```python
from build123d import *

# Parameters (mm, degrees)
BOSS_EXTRUDE1_DEPTH = 2.667
CUT_EXTRUDE1_DEPTH  = 290.953060218


with BuildPart() as part:
    # Sketch1 → Boss-Extrude1 (new body)
    with BuildSketch(Plane(origin=(0, 0, 0), x_dir=(0, 0, -1), z_dir=(1, 0, 0))):
        Polygon((0, 0), (168.275, 0), (251.079, 145), (161.163, 145), align=None)
    extrude(amount=BOSS_EXTRUDE1_DEPTH)

    # Sketch2 → Cut-Extrude1 (cut, through all)
    with BuildSketch(Plane.ZY):
        with BuildLine():
            Line((-38.268496776, -3.7413e-05), (1.603827089, -0.136652983))
            Line((1.603827089, -0.136652983), (-7.656991971, 9.482815094))
            Line((-7.656991971, 9.482815094), (-10.613049229, 9.482815094))
            add(Edge.make_bspline(
                [(-9.096096952, 6.965105301), (-9.056659473, 7.842017541), (-9.649957621, 8.686611456), (-10.613049229, 9.482815094)],
                knots=[0.095003114, 0.095003114, 0.095003114, 0.095003114, 0.122643686, 0.122643686, 0.122643686, 0.122643686], degree=3))
            add(Edge.make_bspline(
                [(-20.479171235, 1.104059742), (-19.78420669, 1.190866413), (-14.294371688, 1.692059126), (-9.186269713, 4.960068489), (-9.096096952, 6.965105301)],
                knots=[0, 0, 0, 0, 0.031803671, 0.095003114, 0.095003114, 0.095003114, 0.095003114], degree=3))
            add(Edge.make_bspline(
                [(-38.268496776, -3.7413e-05), (-29.333639406, -0.001953509), (-20.479171235, 1.104059742)],
                knots=[0, 0, 0, 1, 1, 1], degree=2))
        make_face()
    extrude(amount=-CUT_EXTRUDE1_DEPTH, mode=Mode.SUBTRACT)


solid = part.part
```
For this review, take the finished solid that the model builds, in its own axes (mm). Coordinates: 2 decimals unless noted, no trailing zeros. Write each loop counter-clockwise with the first axis right and the second up, starting at its lowest first coordinate (ties: lowest second). Pieces come first, ordered by that corner, then holes. Notation, with made-up numbers: (33.5, 70) - (57.5, 70) arc R8 ccw to (57.5, 79) - close; hole circle Ø11 at (-15, -22.75). An arc over 180 degrees is marked (long way). Answer in a Markdown table with one row per item. Add a question column.
Q1. For P1, Ø1.5, axis at x = 0.5, z = -138.5, coming from the +Y side, flat-tipped, find the tip position at first contact; note if it passes through.
Q2. For probe 1 along Z at (x, y) = (2.15, 138); probe 2 along Y at (x, z) = (1.75, -211); probe 3 along Y at (x, z) = (1.8, -154), list the stretches that pass through material, from the lowest coordinate up.
Q3. We need section A-A, the plane y = 38. State the section outline as (x, z) points, and give its area (3 significant figures).
Q4. We need section B-B, the plane z = -104. State the section outline as (x, y) points.
Answer list:
| question | item | result |
|---|---|---|
| 1 | P1 | stops at y = 125.28 |
| 2 | probe 1 | z = -247.08 to -153.38 |
| 2 | probe 2 | y = 74.82 to 145 |
| 2 | probe 3 | y = 0 to 138.56 |
| 3 | outline | (0, -189.98) - (2.67, -189.98) - (2.67, -42.24) - (0, -42.24) - close |
| 3 | area | 394 mm2 |
| 4 | outline | (0, 0) - (2.67, 0) - (2.67, 93.57) - (0, 93.57) - close |
